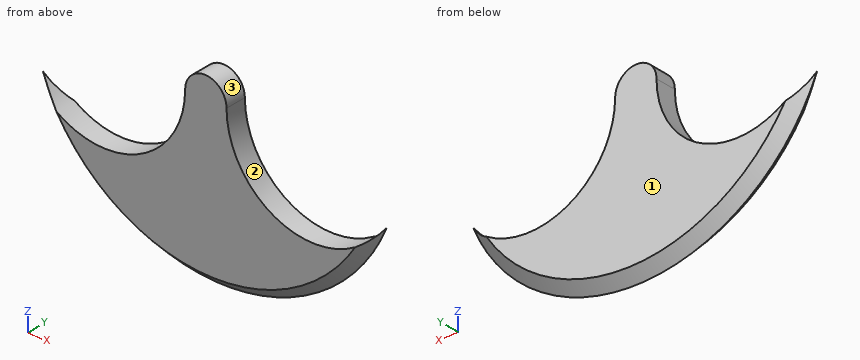
```python
from build123d import *

# Parameters (mm, degrees)
BOSS_EXTRUDE1_DEPTH = 1
CHAMFER1_SIZE       = 1


with BuildPart() as part:
    # Sketch1 → Boss-Extrude1 (new, symmetric)
    with BuildSketch(Plane(origin=(0, 0, 0), x_dir=(1, 0, 0), z_dir=(0, 1, 0))):
        with BuildLine():
            ThreePointArc((16.629831585, 6.888301783), (0, 18), (-16.629831585, 6.888301783))
            ThreePointArc((-16.629831585, 6.888301783), (-7.595646594, 9.851519544), (-2, 2.164784401))
            ThreePointArc((-2, 2.164784401), (0, 0.164784401), (2, 2.164784401))
            ThreePointArc((2, 2.164784401), (7.595646594, 9.851519544), (16.629831585, 6.888301783))
        make_face()
    extrude(amount=BOSS_EXTRUDE1_DEPTH, both=True)

    # Chamfer1
    chamfer1_edges = [part.edges().sort_by_distance(p)[0] for p in [
        (0, -1, -18),
        (0, 1, -18),
    ]]
    chamfer(chamfer1_edges, length=CHAMFER1_SIZE - 0.0001)  # a hair under: the kernel refuses the full size


solid = part.part
```
Could you check a few things on this model? Use its own coordinates, in mm. Face numbers are marked on the shaded views. Coordinates: 2 decimals unless noted, no trailing zeros. Write each loop counter-clockwise with the first axis right and the second up, starting at its lowest first coordinate (ties: lowest second). Pieces come first, ordered by that corner, then holes. Notation, with made-up numbers: (-25, 50) -> (-21, 50) arc R4 ccw to (-21, 57) -> close; hole circle Ø5 at (67.5, -8.75). An arc over 180 degrees is marked (long way). Write item = value, one per line. Start each with the question number.
(1) Will these pins go through, and if not, where does the flat tip stop? pin 1 (1 mm diameter, centred on x = -5, y = 0, fed in from +Z); pin 2 (10 mm diameter, centred on x = 11, z = -5.5, fed in from -Y).
(2) I want a section at B-B (z = -7.5). Give the number of separate pieces and of enclosed holes in the cut face, plus the area to 3 significant figures.
(3) I need wall thicknesses on line 1 (Z direction, x = -14.5, y = -0.5); line 2 (X direction, y = 0.3, z = -15.25); line 3 (Z direction, x = 14, y = -0.7). Which ranges of each line are inside material? Lowest first, please. Write a range as [from, to].
(4) I want a section at C-C (y = 0.55). Please give me the cut outline in (x, z), plus the area to 3 significant figures.
(5) We'd pull the mould along X, two halves only. Please class the marked faces 1, 2 and 3: released by +X, released by -X, zero draft, split by the parting line, or undercut.
Result set:
q1.pin_1 = -8.01
q1.pin_2 = -1
q2.separate_pieces = 3
q2.enclosed_holes = 0
q2.area = 16.1 mm2
q3.line_1 = [-9.8, -8.92]
q3.line_2 = [-8.99, 8.99]
q3.line_3 = [-10.16, -9.23]
q4.outline = (-15.37, -8.27) arc R17.45 ccw to (15.37, -8.27) arc R8.08 cw to (2, -2.16) arc R2 ccw to (-2, -2.16) arc R8.08 cw to start
q4.area = 213 mm2
q5.face_1 = zero draft
q5.face_2 = undercut
q5.face_3 = split by the parting line
